from build123d import *

# Parameters (mm, degrees)
SKETCH1_R           = 2.5
SKETCH1_W           = 97.010301716
SKETCH1_H           = 11.381096849
SKETCH1_H_2         = 9.548114026
SKETCH1_W_2         = 16.423850042
SKETCH1_H_3         = 16.534248646
SKETCH1_W_3         = 21.691877415
SKETCH1_H_4         = 25.100601008
BOSS_EXTRUDE1_DEPTH = 5


with BuildPart() as part:
    # Sketch1 → Boss-Extrude1 (new body)
    with BuildSketch(Plane.XY):
        Polygon((-75, -75), (-52.738744268, -75), (-52.738744268, -70), (-32.738744268, -70), (-32.738744268, -75), (21.360897281, -75), (21.360897281, -70), (41.360897281, -70), (41.360897281, -75), (75, -75), (75, -60.464153422), (70, -60.464153422), (70, -40.464153422), (75, -40.464153422), (75, -13.109084485), (70, -13.109084485), (70, 6.890915515), (75, 6.890915515), (75, 37.435704121), (70.001007164, 37.335351613), (70.001007164, 57.335351613), (75, 57.435704121), (75, 75), (41.360897281, 75), (41.360897281, 70), (21.360897281, 70), (21.360897281, 75), (-32.738744268, 75), (-32.738744268, 70), (-52.738744268, 70), (-52.738744268, 75), (-75, 75), (-75, 57.435704121), (-70.001007164, 57.335351613), (-70.001007164, 37.335351613), (-75, 37.435704121), (-75, 6.890915515), (-70, 6.890915515), (-70, -13.109084485), (-75, -13.109084485), (-75, -40.464153422), (-70, -40.464153422), (-70, -60.464153422), (-75, -60.464153422), align=None)
        Circle(SKETCH1_R, mode=Mode.SUBTRACT)
        with Locations((0, 26.4204034)):
            Rectangle(SKETCH1_W, SKETCH1_H, mode=Mode.SUBTRACT)
        with Locations((0, -23.814174359)):
            Rectangle(SKETCH1_W, SKETCH1_H_2, mode=Mode.SUBTRACT)
        with Locations((-30.010920628, 0)):
            Rectangle(SKETCH1_W_2, SKETCH1_H_3, mode=Mode.SUBTRACT)
        with Locations((32.895523873, 2.888698347)):
            Rectangle(SKETCH1_W_3, SKETCH1_H_4, mode=Mode.SUBTRACT)
    extrude(amount=BOSS_EXTRUDE1_DEPTH)


solid = part.part
Could you check a few things on this model? Use its own coordinates, in mm. A direction names the side the tool comes from. Round coordinates to 2 decimals unless told otherwise and drop trailing zeros. Order: outer loops, then holes, each group sorted by start corner. A loop starts at its lowest first (then second) coordinate and runs counter-clockwise, first axis right, second up.
(1) Imagine slicing it at C-C (x = 0). Write out the boundary of the cut face in (y, z), plus the area to 3 significant figures.
Response values:
outline: (-75, 0) - (-28.59, 0) - (-28.59, 5) - (-75, 5) - close; (-19.04, 0) - (-2.5, 0) - (-2.5, 5) - (-19.04, 5) - close; (2.5, 0) - (20.73, 0) - (20.73, 5) - (2.5, 5) - close; (32.11, 0) - (75, 0) - (75, 5) - (32.11, 5) - close
area: 620 mm2
(2) I'm going to push flat-ended pins straight in: pin 1 (2.5 mm diameter, centred on y = 0.5, z = 1.5, fed in from -X); pin 2 (1.5 mm diameter, centred on y = -2.5, z = 1, fed in from +X). Where does each tip first touch, or does it pass through?
Response values:
pin 1: stops at x = -70
pin 2: stops at x = 70
(3) If we mould it in two halves opening along X, with no side actions, what happens to faces 1 (the flat face through (-32.739, 73, 2)), 2 (the flat face through (-75, -68, 2)), 3 (the flat face through (-72, -13.109, 2)), 4 (the flat face through (75, -27, 2))? For each: released by +X, released by -X, zero draft, split by the parting line, or undercut.
Response values:
face 1: undercut
face 2: released by -X
face 3: zero draft
face 4: released by +X
(4) Please list where these lines run through material, in increasing order: line 1 along Y through (x, z) = (0, 4); line 2 along Y through (x, z) = (18, 0.65); line 3 along Y through (x, z) = (-25.5, 3.4).
Response values:
line 1: y = -75 to -28.59, -19.04 to -2.5, 2.5 to 20.73, 32.11 to 75
line 2: y = -75 to -28.59, -19.04 to 20.73, 32.11 to 75
line 3: y = -75 to -28.59, -19.04 to -8.27, 8.27 to 20.73, 32.11 to 75
(5) Imagine slicing it at D-D (x = -18). Write out the boundary of the cut face in (y, z), plus the area to 3 significant figures.
Response values:
outline: (-75, 0) - (-28.59, 0) - (-28.59, 5) - (-75, 5) - close; (-19.04, 0) - (20.73, 0) - (20.73, 5) - (-19.04, 5) - close; (32.11, 0) - (75, 0) - (75, 5) - (32.11, 5) - close
area: 645 mm2
(6) Imagine slicing it at B-B (x = -41). Write out the boundary of the cut face in (y, z), plus the area to 3 significant figures.
Response values:
outline: (-70, 0) - (-28.59, 0) - (-28.59, 5) - (-70, 5) - close; (-19.04, 0) - (20.73, 0) - (20.73, 5) - (-19.04, 5) - close; (32.11, 0) - (70, 0) - (70, 5) - (32.11, 5) - close
area: 595 mm2
(7) Imagine slicing it at A-A (y = 0). Write out the boundary of the cut face in (x, z), plus the area to 3 significant figures.
Response values:
outline: (-70, 0) - (-38.22, 0) - (-38.22, 5) - (-70, 5) - close; (-21.8, 0) - (-2.5, 0) - (-2.5, 5) - (-21.8, 5) - close; (2.5, 0) - (22.05, 0) - (22.05, 5) - (2.5, 5) - close; (43.74, 0) - (70, 0) - (70, 5) - (43.74, 5) - close
area: 484 mm2
(8) Which directions (+Z, -Z, +X, -X, +Y, -Y) give clear straight access to the entire face, cutting with the end or side of a thin tool? Please do faces 5 (the flat face through (21.361, -73, 2)), 6 (the flat face through (72, -40.464, 2)), 7 (the flat face through (-73, -40.464, 2)), 8 (the flat face through (-52.739, 72, 2)), 9 (the flat face through (-1, -28.588, 2)).
Response values:
face 5: +Z, -Z, -Y
face 6: +Z, -Z, +X
face 7: +Z, -Z, -X
face 8: +Z, -Z, +Y
face 9: +Z, -Z
